from build123d import *

# Parameters (mm, degrees)
BOSS_EXTRUDE1_DEPTH = 2.5
SKETCH2_R           = 1.5
CUT_EXTRUDE1_DEPTH  = 5


with BuildPart() as part:
    # Sketch1 → Boss-Extrude1 (new, symmetric)
    with BuildSketch(Plane.XY):
        with BuildLine():
            Line((-3.25, 0), (3.25, 0))
            Line((3.25, 0), (4.25, 1))
            Line((4.25, 1), (4.603553391, 0.646446609))
            Line((4.603553391, 0.646446609), (3.603553391, -0.353553391))
            ThreePointArc((3.603553391, -0.353553391), (3.441341716, -0.461939766), (3.25, -0.5))
            Line((3.25, -0.5), (-3.25, -0.5))
            ThreePointArc((-3.25, -0.5), (-3.441341716, -0.461939766), (-3.603553391, -0.353553391))
            Line((-3.603553391, -0.353553391), (-4.603553391, 0.646446609))
            Line((-4.603553391, 0.646446609), (-4.25, 1))
            Line((-4.25, 1), (-3.25, 0))
        make_face()
    extrude(amount=BOSS_EXTRUDE1_DEPTH, both=True)

    # Sketch2 → Cut-Extrude1 (cut)
    with BuildSketch(Plane.XZ.offset(0.5)):
        with Locations(Location((0, 0, 0), (0, 0, 270))):
            Circle(SKETCH2_R)
    extrude(amount=-CUT_EXTRUDE1_DEPTH, mode=Mode.SUBTRACT)


solid = part.part
Check sheet for the modelled part. Datum: model origin and axes. Units: mm. A direction names the side the tool comes from. Give positions to 0.01 mm unless a question says otherwise; leave off trailing zeros. Loops run counter-clockwise (first coordinate to the right, second up) from the corner with the lowest first, then second, coordinate; pieces in that order, holes last. Notation, with made-up numbers: M -32.75,18.25 L 13.25,18.25 A22 ccw 13.25,53.25 Z; hole C 69,83.25 d2. An arc over 180 degrees is marked long. Return JSON: item names as keys, results as strings. Group by question number.
1. Thickness scan on L1, parallel to X at y = 0.4, z = -2.15; L2, parallel to X at y = 0.1, z = -1.8; L3, parallel to Y at x = 0.5, z = -1.5. Record the ranges inside material, lowest first.
2. Mould release check, pull along Z, two halves, no side actions. Record for faces 1 (the cylindrical face through (0.45, -0.25, -1.43)), 2 (the flat face through (0, -0.5, 2)), 3 (the flat face through (0.1, -0.2, -2.5)): released by +Z, released by -Z, zero draft, split by the parting line, or undercut.
3. Cross-section at C-C on y = 0.8. Record the boundary of the cut face in (x, z), plus the area to 3 significant figures.
4. Cross-section at D-D on z = 1.2. Record the boundary of the cut face in (x, y).
5. Go/stop test with flat-tipped pins: pin 1 (1.8 mm diameter, centred on x = 0, z = 0, fed in from -Y); pin 2 (2.5 mm diameter, centred on x = -0.5, z = 0.5, fed in from +Y). Record where each tip stops, or that it passes through.
6. Tool access check on faces 4 (the flat face through (0, 0, 2)), 5 (the flat face through (-4.097, 0.139, 0.035)). Record the directions out of +Z, -Z, +X, -X, +Y, -Y that give a thin tool (end or side, any length) a straight path to the whole face; none if there is none.
7. Cross-section at A-A on z = 0. Record the boundary of the cut face in (x, y).
8. Cross-section at B-B on x = 0. Record the boundary of the cut face in (y, z), plus the area to 3 significant figures.
Return value:
{
 "1": {"L1": "-4.36 to -3.65, 3.65 to 4.36", "L2": "-4.06 to -3.35, 3.35 to 4.06", "L3": "-0.5 to 0"},
 "2": {"face 1": "undercut", "face 2": "zero draft", "face 3": "released by -Z"},
 "3": {"outline": "M -4.45,-2.5 L -4.05,-2.5 L -4.05,2.5 L -4.45,2.5 Z; M 4.05,-2.5 L 4.45,-2.5 L 4.45,2.5 L 4.05,2.5 Z", "area": "4.00 mm^2"},
 "4": {"outline": "M -4.6,0.65 L -3.6,-0.35 A0.5 ccw -3.25,-0.5 L -0.9,-0.5 L -0.9,0 L -3.25,0 L -4.25,1 Z; M 0.9,-0.5 L 3.25,-0.5 A0.5 ccw 3.6,-0.35 L 4.6,0.65 L 4.25,1 L 3.25,0 L 0.9,0 Z"},
 "5": {"pin 1": "through", "pin 2": "y = 0"},
 "6": {"face 4": "+Z, -Z, +Y", "face 5": "+Z, -Z, -X, -Y"},
 "7": {"outline": "M -4.6,0.65 L -3.6,-0.35 A0.5 ccw -3.25,-0.5 L -1.5,-0.5 L -1.5,0 L -3.25,0 L -4.25,1 Z; M 1.5,-0.5 L 3.25,-0.5 A0.5 ccw 3.6,-0.35 L 4.6,0.65 L 4.25,1 L 3.25,0 L 1.5,0 Z"},
 "8": {"outline": "M -0.5,-2.5 L 0,-2.5 L 0,-1.5 L -0.5,-1.5 Z; M -0.5,1.5 L 0,1.5 L 0,2.5 L -0.5,2.5 Z", "area": "1.00 mm^2"}
}
